Autodesk Inventor part; units mm, degrees
ref_plane "Arbeitsebene2" through (23.1342, 37.0359, 54) normal (0, 0, 1) x (0.8192, 0.5736, 0)
ref_plane "YZ Plane" through (0, 0, 0) normal (1, 0, 0) x (0, 1, 0)
ref_plane "XZ Plane" through (0, 0, 0) normal (0, 1, 0) x (-1, 0, 0)
ref_plane "Arbeitsebene1" through (0, 0, 0) normal (0, 0, 1) x (1, 0, 0)
sketch "Skizze1" plane through (0, 0, 0) normal (0, 0, 1) x (1, 0, 0)
  circle A0 centre (37.75, -58.75) radius 1.4
  circle A1 centre (37.75, 58.75) radius 1.4
  circle A2 centre (-37.75, 58.75) radius 1.4
  circle A3 centre (-37.75, -58.75) radius 1.4
  circle A4 centre (-28.35, -47.25) radius 8
  circle A5 centre (-28.35, -28.35) radius 8
  circle A6 centre (-28.35, -9.45) radius 8
  circle A7 centre (-28.35, 9.45) radius 8
  circle A8 centre (-28.35, 28.35) radius 8
  circle A9 centre (-28.35, 47.25) radius 8
  circle A10 centre (-9.45, -47.25) radius 8
  circle A11 centre (-9.45, -28.35) radius 8
  circle A12 centre (-9.45, -9.45) radius 8
  circle A13 centre (-9.45, 9.45) radius 8
  circle A14 centre (-9.45, 28.35) radius 8
  circle A15 centre (-9.45, 47.25) radius 8
  circle A16 centre (9.45, -47.25) radius 8
  circle A17 centre (9.45, -28.35) radius 8
  circle A18 centre (9.45, -9.45) radius 8
  circle A19 centre (9.45, 9.45) radius 8
  circle A20 centre (9.45, 28.35) radius 8
  circle A21 centre (9.45, 47.25) radius 8
  circle A22 centre (28.35, -47.25) radius 8
  circle A23 centre (28.35, -28.35) radius 8
  circle A24 centre (28.35, -9.45) radius 8
  circle A25 centre (28.35, 9.45) radius 8
  circle A26 centre (28.35, 28.35) radius 8
  arc A27 (37.75, -63.75) -> (42.75, -58.75) centre (37.75, -58.75) ccw
  line L0 (42.75, -58.75) -> (42.75, 58.75)
  arc A28 (42.75, 58.75) -> (37.75, 63.75) centre (37.75, 58.75) ccw
  line L1 (37.75, 63.75) -> (-37.75, 63.75)
  arc A29 (-37.75, 63.75) -> (-42.75, 58.75) centre (-37.75, 58.75) ccw
  line L2 (-42.75, 58.75) -> (-42.75, -58.75)
  arc A30 (-42.75, -58.75) -> (-37.75, -63.75) centre (-37.75, -58.75) ccw
  line L3 (-37.75, -63.75) -> (37.75, -63.75)
  circle A31 centre (28.35, 47.25) radius 8
  line L4 (41.25, 58.75) -> (41.25, -58.75)
  arc A32 (37.75, -62.25) -> (41.25, -58.75) centre (37.75, -58.75) ccw
  line L5 (37.75, -62.25) -> (-37.75, -62.25)
  arc A33 (-41.25, -58.75) -> (-37.75, -62.25) centre (-37.75, -58.75) ccw
  line L6 (-41.25, -58.75) -> (-41.25, 58.75)
  arc A34 (-37.75, 62.25) -> (-41.25, 58.75) centre (-37.75, 58.75) ccw
  line L7 (-37.75, 62.25) -> (37.75, 62.25)
  arc A35 (41.25, 58.75) -> (37.75, 62.25) centre (37.75, 58.75) ccw
  line L8 (-34.75, 62.25) -> (-34.75, 55.75)
  line L9 (-34.75, 55.75) -> (-41.25, 55.75)
  line L10 (-32.5541, -62.25) -> (-32.5541, -54.8048)
  line L11 (-32.5541, -54.8048) -> (-41.25, -54.8048)
  line L12 (41.25, 55.25) -> (34.25, 55.25)
  line L13 (34.25, 55.25) -> (34.25, 62.25)
  line L14 (31.25, -62.25) -> (24.25, -62.25)
  line L15 (24.25, -62.25) -> (24.25, -55.25)
  line L16 (24.25, -55.25) -> (31.25, -55.25)
  line L17 (31.25, -55.25) -> (31.25, -62.25)
  circle A36 centre (28.25, -59.25) radius 1.4
  point P0 (0, 0)
  point P1 (24.25, -62.25)
  dimension "d0" = 1.5
  dimension "d1" = 3
  dimension "d2" = 3
  dimension "d5" = 7
  dimension "d6" = 7
  dimension "d7" = 7
  dimension "d8" = 7
  dimension "d9" = 10
  dimension "d10" = 2.8
ref_plane "Arbeitsebene2" through (23.1342, 37.0359, 54) normal (0, 0, 1) x (0.8192, 0.5736, 0)
extrude "Extrusion1" add sketch "Skizze1" along normal blind 55 contours L16 L17 L5 L15 | L5 A33 L6 L11 L10 | L12 L13 L7 A35 L4 | L6 A34 L7 L8 L9 | L3 A30 L2 A29 L1 A28 L0 A27
fillet "Rundung1" radius 2 13 edges at (-32.5541, -54.8048, 27.5) (-41.25, -54.8048, 27.5) (-32.5541, -62.25, 27.5) (24.25, -62.25, 27.5) (24.25, -55.25, 27.5) (31.25, -55.25, 27.5) (31.25, -62.25, 27.5) (41.25, 55.25, 27.5) (34.25, 55.25, 27.5) (34.25, 62.25, 27.5) (-34.75, 55.75, 27.5) (-41.25, 55.75, 27.5) (-34.75, 62.25, 27.5)
sketch "Skizze4" plane through (42.75, -58.75, 0) normal (1, 0, 0) x (0, 0, -1)
  line L0 (-43.7633, 6.3718) -> (-13.7057, 6.3718) construction
  line L1 (0, 5.9452) -> (-55, 5.9452)
  line L2 (-43.7633, 3.3718) -> (-13.7057, 3.3718)
  line L3 (-13.7057, 9.3718) -> (-43.7633, 9.3718)
  arc A0 (-43.7633, 9.3718) -> (-43.7633, 3.3718) centre (-43.7633, 6.3718) ccw
  arc A1 (-13.7057, 3.3718) -> (-13.7057, 9.3718) centre (-13.7057, 6.3718) ccw
  point P0 (0, 58.75)
  point P1 (-36.8275, 7.2035)
  point P2 (-36.1925, 26.1035)
  point P3 (-36.1925, 45.0035)
  point P4 (-36.1925, 63.9035)
  point P5 (-36.1925, 82.8035)
  point P6 (-36.1925, 101.7035)
  point P7 (-28.7345, 6.3718)
  dimension "d29" = 6
extrude "Extrusion4" cut sketch "Skizze4" against normal blind 55
pattern_linear "Rechteckige Anordnung2" count 6 spacing 18.9 along (0, 1, 0) of "Extrusion4"
ref_plane "Arbeitsebene3" through (0, -58.75, 0) normal (1, 0, 0) x (0, 0, -1)
ref_plane "Arbeitsebene4" through (-37.75, 0, 0) normal (0, 1, 0) x (1, 0, 0)
sketch "Skizze5" plane through (-37.75, 63.75, 0) normal (0, 1, 0) x (1, 0, 0)
  line L0 (75.5, 0) -> (0, 0)
  line L1 (0, 0) -> (0, -55)
  line L2 (75.5, -55) -> (0, -55)
  line L3 (75.5, 0) -> (75.5, -55)
  line L4 (60.25, -42.5) -> (15.25, -42.5)
  line L5 (15.25, -42.5) -> (15.25, -12.5)
  line L6 (15.25, -12.5) -> (60.25, -12.5)
  line L7 (60.25, -12.5) -> (60.25, -42.5)
  line L8 (60.25, -42.5) -> (15.25, -12.5) construction
  line L9 (15.25, -42.5) -> (60.25, -12.5) construction
  point P0 (37.75, 0)
  point P1 (52.5946, -34.1859)
  point P2 (37.75, -27.5)
  dimension "d35" = 45
  dimension "d36" = 30
hole "Bohrung1" at (22.5, 63.75, 42.5) at (-22.5, 63.75, 42.5) at (-22.5, 63.75, 12.5) at (22.5, 63.75, 12.5) direction (0, -1, 0) diameter 2.8 end through all
ref_plane "Arbeitsebene5" through (-37.75, 0, 0) normal (0, 1, 0) x (1, 0, 0)
properties part number "Omniscope_sidewalls_v0"
The model under review builds one solid part; all positions refer to its coordinate system, in mm. A direction names the side the tool comes from. Coordinates: 2 decimals unless noted, no trailing zeros. Write each loop counter-clockwise with the first axis right and the second up, starting at its lowest first coordinate (ties: lowest second). Pieces come first, ordered by that corner, then holes. Notation, with made-up numbers: M -40,47 L -4,47 A14 ccw -4,66 Z; hole C -23,-0.5 d3. An arc over 180 degrees is marked long. Put each result on its own line as item: value.
1) Add section C-C on z = 38.5. State how many separate pieces and enclosed holes the cut face has, then the cut area to 3 significant figures.
Computed:
separate pieces: 6
enclosed holes: 4
area: 740 mm2
2) Add section B-B on y = 29. Give the boundary of the cut face in (x, z).
Computed:
outline: M -42.75,0 L -41.25,0 L -41.25,55 L -42.75,55 Z; M 41.25,0 L 42.75,0 L 42.75,55 L 41.25,55 Z
3) Draft analysis for pull direction Y (two halves, no side actions). For faces 4 (the flat face through (38, 55.25, 27)), 5 (the cylindrical face through (-41.32, 62.25, 27.12)), 6 (the cylindrical face through (-41.25, -62.32, 27.12)), 7 (the flat face through (42.75, -1, 27)), state which applies: released by +Y, released by -Y, zero draft, split by the parting line, or undercut.
Computed:
face 4: undercut
face 5: released by +Y
face 6: released by -Y
face 7: zero draft
4) Clearance check with flat-ended pins moving along their axes: pin 1 Ø4.5 at (x, z) = (-22.5, 42.5) entering from +Y; pin 2 Ø1.6 at (x, z) = (42, 25) entering from -Y. State where each tip first meets the part, or that it passes through.
Computed:
pin 1: stops at y = 63.75
pin 2: stops at y = -62.37
5) Add section A-A on x = -15. Give the boundary of the cut face in (y, z).
Computed:
outline: M -63.75,0 L -62.25,0 L -62.25,55 L -63.75,55 Z; M 62.25,0 L 63.75,0 L 63.75,55 L 62.25,55 Z
6) Wall thickness on probe 1 along X at (y, z) = (-10.5, 41); probe 2 along Z at (x, y) = (-22.5, 62.6); probe 3 along Y at (x, z) = (-7, 38.5): over which ranges is each line inside the solid? List them lowest first. Write a range as [from, to].
Computed:
probe 1: x = [-42.75, -41.25], [41.25, 42.75]
probe 2: z = [0, 11.1], [13.9, 41.1], [43.9, 55]
probe 3: y = [-63.75, -62.25], [62.25, 63.75]
7) For faces 1 (the cylindrical face through (42.01, -52.312, 46.763)), 2 (the flat face through (31.25, -59, 27)), 3 (the flat face through (-42.75, 1, 27)), list the 3-axis set-ups (+Z, -Z, +X, -X, +Y, -Y) from which the entire face can be reached by the end or side of a thin tool; tool diameter is ignored.
Computed:
face 1: +X
face 2: +Z, -Z
face 3: +Z, -Z, -X, +Y, -Y
